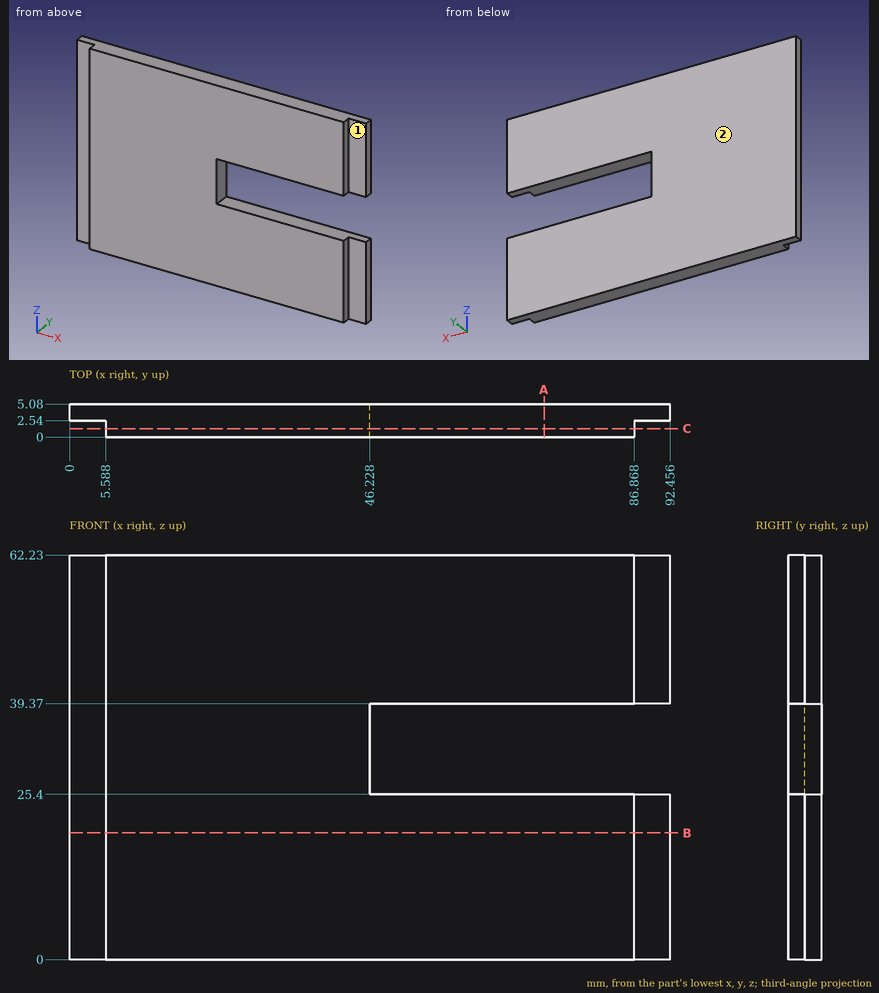
Here's the drawing with two shaded views (mm, measured from the low corner). I have some questions. A direction names the side the tool comes from. Round coordinates to 2 decimals unless told otherwise and drop trailing zeros. Write each loop counter-clockwise with the first axis right and the second up, starting at its lowest first coordinate (ties: lowest second). Pieces come first, ordered by that corner, then holes. Notation, with made-up numbers: M 71.25,-29 L 108.25,-29 A32 cw 108.25,0 Z; hole C 71.25,-21 d3. An arc over 180 degrees is marked long. Write each question's results on one line, items separated by ' | '. Start each with the question number.
1. I need wall thicknesses on L1, parallel to Z at x = 83, y = 4.5; L2, parallel to X at y = 0.8, z = 14.5; L3, parallel to X at y = 2.3, z = 27. Which ranges of each line are inside material? Lowest first, please. Write a range as from..to.
2. I'm going to push flat-ended pins straight in: pin 1 Ø3 at (y, z) = (1, 18.5) entering from -X; pin 2 Ø1.7 at (x, z) = (3, 18) entering from -Y; pin 3 Ø2 at (y, z) = (1.5, 38) entering from +X. Where does each tip first touch, or does it pass through?
3. On a 3-axis mill with a long thin cutter (end or side, diameter ignored), from which of +Z, -Z, +X, -X, +Y, -Y can I reach the whole of each face in a straight line? I mean the marked faces 1 and 2. Say none if no direction works.
4. Imagine slicing it at C-C on y = 1.3. List the corners of the cut face in (x, z) for me.
5. Imagine slicing it at B-B on z = 19.5. List the corners of the cut face in (x, y) for me, and give its area (3 significant figures).
6. Imagine slicing it at A-A on x = 73. List the corners of the cut face in (y, z) for me.
Result sheet:
1) L1: z = 0..25.4, 39.37..62.23 | L2: x = 5.59..86.87 | L3: x = 5.59..46.23
2) pin 1: stops at x = 5.59 | pin 2: stops at y = 2.54 | pin 3: stops at x = 46.23
3) face 1: +Z, -Z, +X, -Y | face 2: +Z, -Z, +X, -X, +Y
4) outline: M 5.59,0 L 86.87,0 L 86.87,25.4 L 46.23,25.4 L 46.23,39.37 L 86.87,39.37 L 86.87,62.23 L 5.59,62.23 Z
5) outline: M 0,2.54 L 5.59,2.54 L 5.59,0 L 86.87,0 L 86.87,2.54 L 92.46,2.54 L 92.46,5.08 L 0,5.08 Z | area: 441 mm^2
6) outline: M 0,0 L 5.08,0 L 5.08,25.4 L 0,25.4 Z; M 0,39.37 L 5.08,39.37 L 5.08,62.23 L 0,62.23 Z
